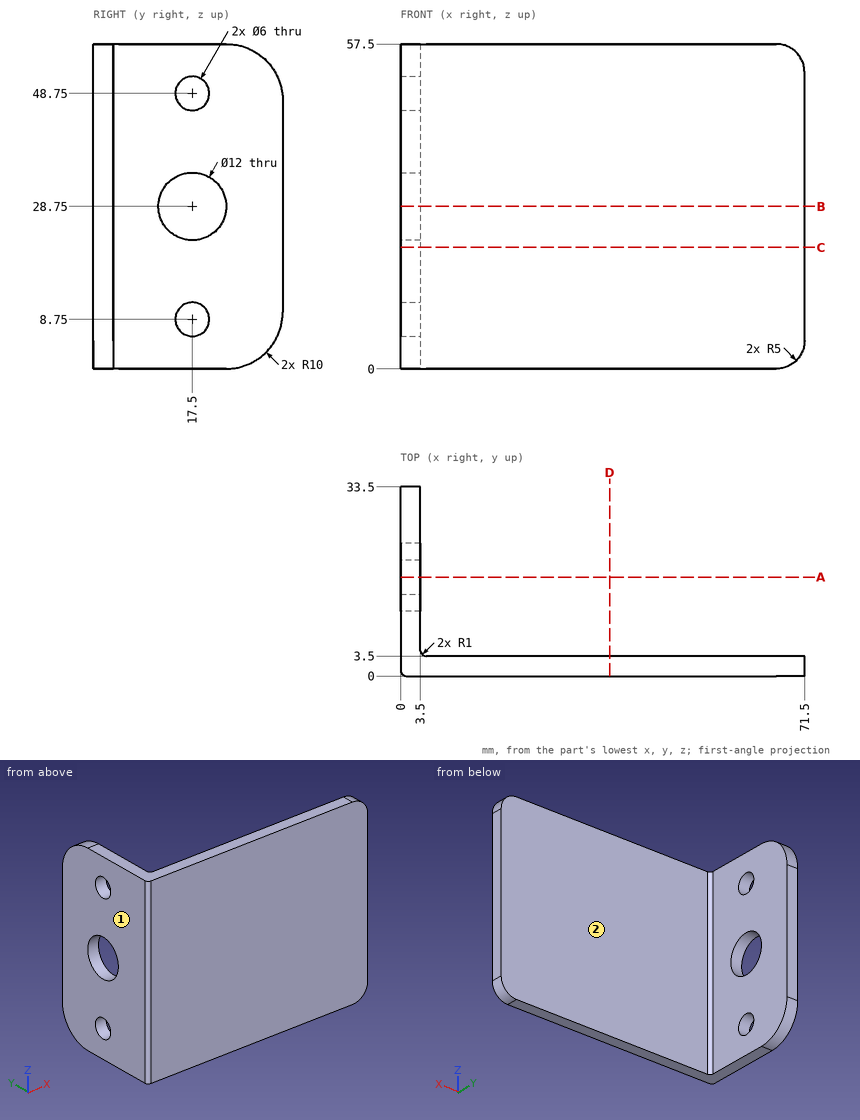
Answer from the drawing. Dimensions are ordinates in mm from the lowest x, y and z of the part. A direction names the side the tool comes from. Coordinates: 2 decimals unless noted, no trailing zeros. Loops run counter-clockwise (first coordinate to the right, second up) from the corner with the lowest first, then second, coordinate; pieces in that order, holes last.
Q1. The part is cut by section B-B on z = 28.75. Write down the section's boundary in (x, y).
Q2. The part is cut by section A-A on y = 17.5. Write down the section's boundary in (x, z), and give its area (3 significant figures).
Q3. Consider probe 1 along Z at (x, y) = (1, 17); probe 2 along X at (y, z) = (18, 18). Determine where each line is inside the solid, lowest interval first.
Q4. Each of these flat-tipped pins is pushed along its axis until it touches: pin 1 Ø14 at (y, z) = (17.5, 28.75) entering from -X; pin 2 Ø10 at (x, y) = (20.5, 10) entering from +Z; pin 3 Ø6 at (y, z) = (17.5, 37) entering from +X; pin 4 Ø3 at (x, z) = (62, 28.5) entering from +Y. Where does it stop, or does it pass through?
Q5. Which of the six approach directions +Z, -Z, +X, -X, +Y, -Y give full straight-line access (tool end or side, diameter ignored) to the marked faces 1 and 2?
Q6. The part is cut by section C-C on z = 21.5. Write down the section's boundary in (x, y), and give its area (3 significant figures).
Q7. The part is cut by section D-D on x = 37. Write down the section's boundary in (y, z).
Results below:
1. outline: (0, 1) arc R1 ccw to (1, 0) - (71.5, 0) - (71.5, 3.5) - (4.5, 3.5) arc R1 cw to (3.5, 4.5) - (3.5, 11.5) - (0, 11.5) - close; (0, 23.5) - (3.5, 23.5) - (3.5, 33.5) - (0, 33.5) - close
2. outline: (0, 0) - (3.5, 0) - (3.5, 5.75) - (0, 5.75) - close; (0, 11.75) - (3.5, 11.75) - (3.5, 22.75) - (0, 22.75) - close; (0, 34.75) - (3.5, 34.75) - (3.5, 45.75) - (0, 45.75) - close; (0, 51.75) - (3.5, 51.75) - (3.5, 57.5) - (0, 57.5) - close
2. area: 117 mm2
3. probe 1: z = 0 to 5.79, 11.71 to 22.77, 34.73 to 45.79, 51.71 to 57.5
3. probe 2: x = 0 to 3.5
4. pin 1: stops at x = 0
4. pin 2: passes through
4. pin 3: stops at x = 3.5
4. pin 4: stops at y = 3.5
5. face 1: +Z, -Z, -X, +Y, -Y
5. face 2: +Z, -Z, +X, +Y
6. outline: (0, 1) arc R1 ccw to (1, 0) - (71.5, 0) - (71.5, 3.5) - (4.5, 3.5) arc R1 cw to (3.5, 4.5) - (3.5, 33.5) - (0, 33.5) - close
6. area: 355 mm2
7. outline: (0, 0) - (3.5, 0) - (3.5, 57.5) - (0, 57.5) - close
